Input: dimensioned drawing with shaded views. Units: mm. Origin: part minimum x, y, z. A direction names the side the tool comes from. Give positions to 0.01 mm unless a question says otherwise; leave off trailing zeros. Loops run counter-clockwise (first coordinate to the right, second up) from the corner with the lowest first, then second, coordinate; pieces in that order, holes last. Notation, with made-up numbers: (63.5, 53) -> (92.5, 53) arc R34 cw to (92.5, 83) -> close; hole circle Ø7 at (32, 74.5). An arc over 180 degrees is marked (long way). One line per question, with ' | ' between items. Start each with the question number.
Item 1: Mould query, pull axis Y, two halves, no side actions, for the marked faces 1, 2 and 3. Classes: released by +Y, released by -Y, zero draft, split by the parting line, or undercut.
Item 2: Section D-D on y = 81.5. Return loops of the section in (x, z), then the cut area to 3 significant figures.
Item 3: Pin query (flat end, axial travel): P1, Ø6, axis at x = 23.5, z = 17, coming from the -Y side; P2, Ø5, axis at x = 20.5, y = 86.5, coming from the -Z side; P3, Ø6, axis at y = 45, z = 31.5, coming from the +X side; P4, Ø2, axis at y = 43.5, z = 21, coming from the -X side. Return the tip coordinate at first contact, or that it passes through.
Item 4: Material intervals for line 1 along Y through (x, z) = (50, 3.35); line 2 along Y through (x, z) = (50, 8); line 3 along Z through (x, y) = (38, 81), sorted ascending. Write a range as [from, to].
Item 5: Section A-A on x = 50. Return loops of the section in (y, z).
Item 6: Set-up query: the marked faces 4 and 5. Return all of +Z, -Z, +X, -X, +Y, -Y with unobstructed straight access to the full face (end or side cutting, diameter ignored); none if empty.
Item 7: Section C-C on z = 24.5. Return loops of the section in (x, y), then the cut area to 3 significant figures.
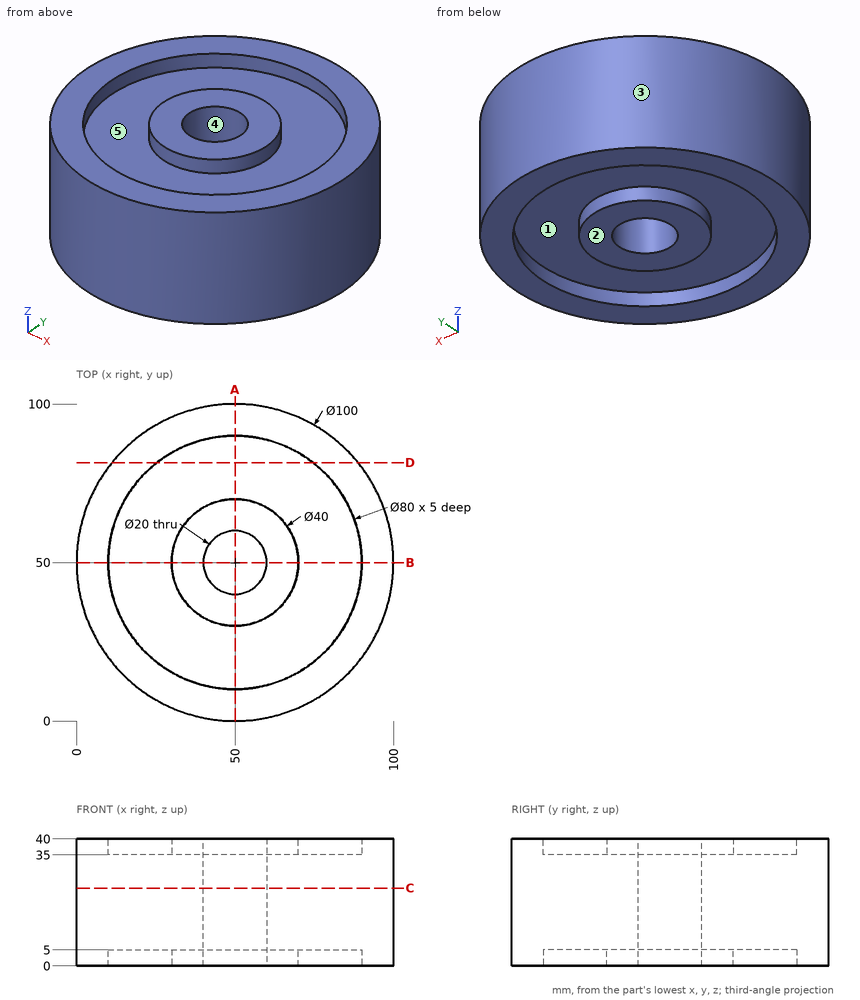
Result sheet:
1) face 1: undercut | face 2: zero draft | face 3: split by the parting line
2) outline: (11.17, 0) -> (25.35, 0) -> (25.35, 5) -> (74.65, 5) -> (74.65, 0) -> (88.83, 0) -> (88.83, 40) -> (74.65, 40) -> (74.65, 35) -> (25.35, 35) -> (25.35, 40) -> (11.17, 40) -> close | area: 2,610 mm²
3) P1: stops at y = 5.87 | P2: stops at z = 0 | P3: stops at x = 99.96 | P4: stops at x = 0.3
4) line 1: y = [0, 10], [30, 40], [60, 70], [90, 100] | line 2: y = [0, 40], [60, 100] | line 3: z = [5, 35]
5) outline: (0, 0) -> (10, 0) -> (10, 5) -> (30, 5) -> (30, 0) -> (40, 0) -> (40, 40) -> (30, 40) -> (30, 35) -> (10, 35) -> (10, 40) -> (0, 40) -> close; (60, 0) -> (70, 0) -> (70, 5) -> (90, 5) -> (90, 0) -> (100, 0) -> (100, 40) -> (90, 40) -> (90, 35) -> (70, 35) -> (70, 40) -> (60, 40) -> close
6) face 4: +Z, -Z | face 5: +Z
7) outline: circle Ø100 at (50, 50); hole circle Ø20 at (50, 50) | area: 7,540 mm²
